Could you check a few things on this model? Use its own coordinates, in mm. A direction names the side the tool comes from. Coordinates: 2 decimals unless noted, no trailing zeros. Order: outer loops, then holes, each group sorted by start corner. A loop starts at its lowest first (then second) coordinate and runs counter-clockwise, first axis right, second up. Notation, with made-up numbers: (18, 69.25) - (62, 69.25) arc R18 cw to (62, 82.25) - close; hole circle Ø3 at (28.5, 74.25). An arc over 180 degrees is marked (long way). One line per item, written item: value.
from build123d import *

# Parameters (mm, degrees)
PAD_DEPTH            = 20
POLARPATTERN_COUNT   = 4
FILLET_R             = 1.5
CHAMFER_SIZE         = 1.5
BODY_PLACEMENT_ANGLE = 270


with BuildPart() as part:
    # Sketch → Pad (new body)
    with BuildSketch(Plane.XZ):
        with BuildLine():
            Line((0, 3.9), (2.627208, 3.9))
            Line((2.627208, 3.9), (6.927208, 8.2))
            Line((6.927208, 8.2), (3.1, 8.2))
            Line((3.1, 8.2), (3.1, 10))
            Line((3.1, 10), (10, 10))
            Line((10, 10), (10, 3.1))
            Line((10, 3.1), (8.2, 3.1))
            Line((8.2, 3.1), (8.2, 6.927208))
            Line((3.9, 2.627208), (8.2, 6.927208))
            Line((3.9, 2.627208), (3.9, 0))
            Line((2.5, 0), (3.9, 0))
            ThreePointArc((2.5, 0), (1.767767, 1.767767), (0, 2.5))
            Line((0, 3.9), (0, 2.5))
        make_face()
    pad = extrude(amount=PAD_DEPTH)

    # PolarPattern: Pad ×4 about axis
    polarpattern_axis = Axis((0, 0, 0), (0, -1, 0))
    for i in range(1, POLARPATTERN_COUNT):
        add(pad.rotate(polarpattern_axis, i * 360 / POLARPATTERN_COUNT))

    # Fillet
    fillet_edges = [part.edges().sort_by_distance(p)[0] for p in [
        (-10, -10, 10),
        (10, -10, 10),
        (10, -10, -10),
        (-10, -10, -10),
    ]]
    fillet(fillet_edges, radius=FILLET_R)

    # Chamfer
    chamfer_edges = [part.edges().sort_by_distance(p)[0] for p in [
        (3.1, -10, 10),
        (-3.1, -10, 10),
        (-10, -10, 3.1),
        (-10, -10, -3.1),
        (-3.1, -10, -10),
        (10, -10, -3.1),
        (3.1, -10, -10),
        (10, -10, 3.1),
    ]]
    chamfer(chamfer_edges, length=CHAMFER_SIZE)


with BuildPart() as part_1:
    # Body placement: moved
    add(part.part.rotate(Axis((0, 0, 0), (1, 0, 0)), BODY_PLACEMENT_ANGLE))


solid = part_1.part
Item 1: I want a section at C-C on y = -5. Please give me the cut outline in (x, z).
Conclusion:
outline: (-10, 0) - (-8.2, 0) - (-8.2, 20) - (-10, 20) - close; (-6.27, 0) - (-3.73, 0) - (-3.73, 20) - (-6.27, 20) - close; (3.73, 0) - (6.27, 0) - (6.27, 20) - (3.73, 20) - close; (8.2, 0) - (10, 0) - (10, 20) - (8.2, 20) - close
Item 2: If I drill on probe 1 along X at (y, z) = (3.75, 3.25); probe 2 along X at (y, z) = (-6, 7); probe 3 along X at (y, z) = (4.75, 10.5), over which ranges is the centre line in solid material (lowest first)?
Conclusion:
probe 1: -9.15 to -8.2, -5.02 to 5.02, 8.2 to 9.15
probe 2: -10 to -8.2, -7.27 to -4.73, 4.73 to 7.27, 8.2 to 10
probe 3: -10 to -8.2, -6.02 to -3.48, 3.48 to 6.02, 8.2 to 10
Item 3: Thinking about a two-plate mould opening in Y: for faces 6 (the face through (-3.9, -9.3, 9.9)), 7 (the face through (-3.9, 9.3, 9.9)), 8 (the face through (-8.2, -5, 10)), 9 (the face through (3.9, 0, 10)), which applies, pulls with the +Y half, pulls with the -Y half, needs draft (parallel to the pull), parting line crosses it, or undercut?
Conclusion:
face 6: pulls with the -Y half
face 7: pulls with the +Y half
face 8: undercut
face 9: undercut
Item 4: For faces 1 (the face through (2, -2, 0)), 2 (the face through (3.8, -9.2, 9.9)), 3 (the face through (-8.2, 5, 10)), 4 (the face through (-9.57, -9.55, 10.14)), 5 (the face through (-9.2, -3.8, 9.9)), which set-ups out of +Z, -Z, +X, -X, +Y, -Y let a thin tool reach every point of the face, with its end or its side?
Conclusion:
face 1: -Z, +X, -X, +Y, -Y
face 2: +Z, -Z, -Y
face 3: +Z, -Z
face 4: +Z, -Z, -X, -Y
face 5: +Z, -Z, -X
Item 5: I want a section at A-A on y = 2. Please give me the cut outline in (x, z).
Conclusion:
outline: (-3.9, 0) - (-1.5, 0) - (-1.5, 20) - (-3.9, 20) - close; (1.5, 0) - (3.9, 0) - (3.9, 20) - (1.5, 20) - close
Item 6: I want a section at D-D on y = -1. Please give me the cut outline in (x, z).
Conclusion:
outline: (-3.9, 0) - (-2.29, 0) - (-2.29, 20) - (-3.9, 20) - close; (2.29, 0) - (3.9, 0) - (3.9, 20) - (2.29, 20) - close
Item 7: I want a section at B-B on x = 3.5. Please give me the cut outline in (y, z).
Conclusion:
outline: (-8.9, 0) - (-8.2, 0) - (-8.2, 20) - (-8.9, 20) - close; (-4.77, 0) - (4.77, 0) - (4.77, 20) - (-4.77, 20) - close; (8.2, 0) - (8.9, 0) - (8.9, 20) - (8.2, 20) - close
Item 8: I'm going to push flat-ended pins straight in: pin 1 Ø8 at (x, z) = (4.5, 6) entering from +Y; pin 2 Ø4 at (x, z) = (1, 10) entering from +Y; pin 3 Ø1 at (y, z) = (-0.5, 17) entering from +X; pin 4 Ø6 at (y, z) = (-1, 12.5) entering from -X. Where does each tip first touch, or does it pass through?
Conclusion:
pin 1: y = 10
pin 2: y = 4.27
pin 3: x = 3.9
pin 4: x = -9.4
